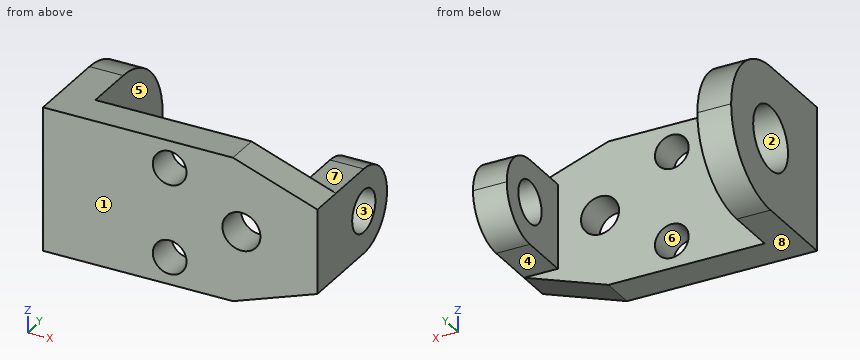
```python
from build123d import *

# Parameters (mm, degrees)
SKETCH1_R           = 4
SKETCH1_R_2         = 4.5
SKETCH1_W           = 8
SKETCH1_H           = 34
SKETCH1_H_2         = 20
BOSS_EXTRUDE1_DEPTH = 8
SKETCH1_4_W         = 8
SKETCH1_4_H         = 34
BOSS_EXTRUDE2_DEPTH = 37
SKETCH1_5_W         = 8
SKETCH1_5_H         = 20
BOSS_EXTRUDE3_DEPTH = 30
SKETCH4_R           = 5
CUT_EXTRUDE1_DEPTH  = 8
SKETCH5_R           = 7.5
CUT_EXTRUDE2_DEPTH  = 71.049982156


with BuildPart() as part:
    # Sketch1 → Boss-Extrude1 (new body)
    # profile 1 of 3: a face of its own
    with BuildSketch(Plane(origin=(0, 0, 0), x_dir=(1, 0, 0), z_dir=(0, 1, 0))):
        Polygon((8, 17), (8, -17), (45, -17), (65, -10), (57, -10), (57, 10), (65, 10), (45, 17), align=None)
        with Locations(Location((30, -10.563020066, 0), (0, 0, 270))):
            Circle(SKETCH1_R, mode=Mode.SUBTRACT)
        with Locations(Location((30, 10.563020066, 0), (0, 0, 270))):
            Circle(SKETCH1_R, mode=Mode.SUBTRACT)
        with Locations(Location((47, 0, 0), (0, 0, 270))):
            Circle(SKETCH1_R_2, mode=Mode.SUBTRACT)
    # profile 2 of 3: a face of its own
    with BuildSketch(Plane(origin=(0, 0, 0), x_dir=(1, 0, 0), z_dir=(0, 1, 0))):
        with Locations((4, 0)):
            Rectangle(SKETCH1_W, SKETCH1_H)
    # profile 3 of 3: a face of its own
    with BuildSketch(Plane(origin=(0, 0, 0), x_dir=(1, 0, 0), z_dir=(0, 1, 0))):
        with Locations((61, 0)):
            Rectangle(SKETCH1_W, SKETCH1_H_2)
    extrude(amount=BOSS_EXTRUDE1_DEPTH)

    # Sketch1<4> → Boss-Extrude2 (add)
    with BuildSketch(Plane(origin=(0, 0, 0), x_dir=(1, 0, 0), z_dir=(0, 1, 0))):
        with Locations((4, 0)):
            Rectangle(SKETCH1_4_W, SKETCH1_4_H)
    extrude(amount=BOSS_EXTRUDE2_DEPTH)

    # Sketch1<5> → Boss-Extrude3 (add)
    with BuildSketch(Plane(origin=(0, 0, 0), x_dir=(1, 0, 0), z_dir=(0, 1, 0))):
        with Locations((61, 0)):
            Rectangle(SKETCH1_5_W, SKETCH1_5_H)
    extrude(amount=BOSS_EXTRUDE3_DEPTH)

    # Sketch4 → Cut-Extrude1 (cut)
    with BuildSketch(Plane(origin=(65, 0, 0), x_dir=(0, 0, -1), z_dir=(1, 0, 0))):
        with BuildLine():
            ThreePointArc((0, 30), (7.071067812, 27.071067812), (10, 20))
            Line((10, 20), (10, 30))
            Line((10, 30), (0, 30))
        make_face()
        with BuildLine():
            ThreePointArc((-10, 20), (-7.071067812, 27.071067812), (0, 30))
            Line((0, 30), (-10, 30))
            Line((-10, 30), (-10, 20))
        make_face()
        with Locations((0, 20)):
            Circle(SKETCH4_R)
    extrude(amount=-CUT_EXTRUDE1_DEPTH, mode=Mode.SUBTRACT)

    # Sketch5 → Cut-Extrude2 (cut, through all)
    with BuildSketch(Plane(origin=(8, 0, 0), x_dir=(0, 0, -1), z_dir=(1, 0, 0))):
        with BuildLine():
            ThreePointArc((-17, 20), (-12.02081528, 32.02081528), (0, 37))
            Line((0, 37), (-17, 37))
            Line((-17, 37), (-17, 20))
        make_face()
        with BuildLine():
            ThreePointArc((0, 37), (12.02081528, 32.02081528), (17, 20))
            Line((17, 20), (17, 37))
            Line((17, 37), (0, 37))
        make_face()
        with Locations((0, 20)):
            Circle(SKETCH5_R)
    extrude(amount=-CUT_EXTRUDE2_DEPTH, mode=Mode.SUBTRACT)


solid = part.part
```
For this review, take the finished solid that the model builds, in its own axes (mm). Face numbers are marked on the shaded views. A direction names the side the tool comes from. Coordinates: 2 decimals unless noted, no trailing zeros. Loops run counter-clockwise (first coordinate to the right, second up) from the corner with the lowest first, then second, coordinate; pieces in that order, holes last. Notation, with made-up numbers: (57.5, 10) - (116.5, 10) arc R11 cw to (116.5, 28) - close; hole circle Ø7 at (0.5, 5.25). An arc over 180 degrees is marked (long way). Use one line per item in the form item = value. Start each with the question number.
1) Take a section at C-C (y = 6.5). State the section outline as (x, z) points.
2) Take a section at B-B (x = 30). State the section outline as (y, z) points.
3) Draft analysis for pull direction Z (two halves, no side actions). For the marked faces 6, 7 and 8, state which applies: released by +Z, released by -Z, zero draft, split by the parting line, or undercut.
4) For the marked faces 1, 2, 3, 4 and 5, list the 3-axis set-ups (+Z, -Z, +X, -X, +Y, -Y) from which the entire face can be reached by the end or side of a thin tool; tool diameter is ignored.
5) For pin 1 (8 mm diameter, centred on x = 22, z = 2.5, fed in from +Y); pin 2 (6.5 mm diameter, centred on x = 60.5, y = 13, fed in from +Z); pin 3 (4 mm diameter, centred on x = 62, y = 13.5, fed in from -Z); pin 4 (7 mm diameter, centred on x = 47, z = 0, fed in from +Y), all flat-tipped, find the tip position at first contact; note any pin that passes through.
6) Take a section at D-D (x = 60). State the section outline as (y, z) points.
7) Take a section at A-A (x = 47). State the section outline as (y, z) points, plus the area to 3 significant figures.
8) To check wall thickness, follow probe 1 along X at (y, z) = (18, 8.5); probe 2 along Y at (x, z) = (26.5, -13); probe 3 along X at (y, z) = (25.5, -2). State the ranges of each line that lie inside material, in increasing order. Write a range as from..to.
From the geometry:
q1.outline = (0, -17) - (45, -17) - (65, -10) - (65, 10) - (45, 17) - (0, 17) - close; hole circle Ø8 at (30, -10.56); hole circle Ø8 at (30, 10.56); hole circle Ø9 at (47, 0)
q2.outline = (0, -17) - (8, -17) - (8, -14.56) - (0, -14.56) - close; (0, -6.56) - (8, -6.56) - (8, 6.56) - (0, 6.56) - close; (0, 14.56) - (8, 14.56) - (8, 17) - (0, 17) - close
q3.face_6 = undercut
q3.face_7 = released by +Z
q3.face_8 = released by -Z
q4.face_1 = +Z, -Z, +X, -X, -Y
q4.face_2 = -X
q4.face_3 = +X, -X
q4.face_4 = -Z, +X, +Y
q4.face_5 = +Z, -Z, +Y
q5.pin_1 = 8
q5.pin_2 = 10
q5.pin_3 = -10
q5.pin_4 = through
q6.outline = (0, -11.75) - (8, -11.75) - (8, -10) - (20, -10) arc R10 ccw to (20, 10) - (8, 10) - (8, 11.75) - (0, 11.75) - close; hole circle Ø10 at (20, 0)
q7.outline = (0, -16.3) - (8, -16.3) - (8, -4.5) - (0, -4.5) - close; (0, 4.5) - (8, 4.5) - (8, 16.3) - (0, 16.3) - close
q7.area = 189 mm2
q8.probe_1 = 0..8, 57..65
q8.probe_2 = 0..8
q8.probe_3 = 57..65
